Could you check a few things on this model? Use its own coordinates, in mm. A direction names the side the tool comes from. Coordinates: 2 decimals unless noted, no trailing zeros. Loops run counter-clockwise (first coordinate to the right, second up) from the corner with the lowest first, then second, coordinate; pieces in that order, holes last.
from build123d import *

# Parameters (mm, degrees)
SKETCH1_W             = 6.5
SKETCH1_H             = 3.5
BOSS_EXTRUDE1_DEPTH   = 1.6
CHAMFER1_SIZE         = 1
CHAMFER1_SIZE2        = 0.25
CHAMFER1_PART_2_SIZE  = 1
CHAMFER1_PART_2_SIZE2 = 0.25
CHAMFER1_PART_3_SIZE  = 1
CHAMFER1_PART_3_SIZE2 = 0.25
CHAMFER1_PART_4_SIZE  = 1
CHAMFER1_PART_4_SIZE2 = 0.25
CHAMFER2_SIZE         = 0.125
CHAMFER2_SIZE2        = 0.5
EXTRUDE_THIN1_DEPTH   = 1.5
EXTRUDE_THIN2_DEPTH   = 0.35
LPATTERN1_COUNT       = 3
LPATTERN1_PITCH       = 2.3


with BuildPart() as part:
    # Sketch1 → Boss-Extrude1 (new body)
    with BuildSketch(Plane(origin=(0, 0, 0), x_dir=(1, 0, 0), z_dir=(0, 1, 0))):
        Rectangle(SKETCH1_W, SKETCH1_H)
    extrude(amount=BOSS_EXTRUDE1_DEPTH)

    # Chamfer1
    chamfer1_edges = [part.edges().sort_by_distance(p)[0] for p in [
        (3.25, 1.6, 0),
    ]]
    chamfer1_side = [part.faces().sort_by_distance(p)[0] for p in [
        (3.25, 0.8, 0),
    ]]
    chamfer(chamfer1_edges, length=CHAMFER1_SIZE, length2=CHAMFER1_SIZE2, reference=chamfer1_side[0])

    # Chamfer1 part 2
    chamfer1_part_2_edges = [part.edges().sort_by_distance(p)[0] for p in [
        (0, 1.6, -1.75),
    ]]
    chamfer1_part_2_side = [part.faces().sort_by_distance(p)[0] for p in [
        (0, 0.8, -1.75),
    ]]
    chamfer(chamfer1_part_2_edges, length=CHAMFER1_PART_2_SIZE, length2=CHAMFER1_PART_2_SIZE2, reference=chamfer1_part_2_side[0])

    # Chamfer1 part 3
    chamfer1_part_3_edges = [part.edges().sort_by_distance(p)[0] for p in [
        (-3.25, 1.6, 0),
    ]]
    chamfer1_part_3_side = [part.faces().sort_by_distance(p)[0] for p in [
        (-3.25, 0.8, 0),
    ]]
    chamfer(chamfer1_part_3_edges, length=CHAMFER1_PART_3_SIZE, length2=CHAMFER1_PART_3_SIZE2, reference=chamfer1_part_3_side[0])

    # Chamfer1 part 4
    chamfer1_part_4_edges = [part.edges().sort_by_distance(p)[0] for p in [
        (0, 1.6, 1.75),
    ]]
    chamfer1_part_4_side = [part.faces().sort_by_distance(p)[0] for p in [
        (0, 0.8, 1.75),
    ]]
    chamfer(chamfer1_part_4_edges, length=CHAMFER1_PART_4_SIZE, length2=CHAMFER1_PART_4_SIZE2, reference=chamfer1_part_4_side[0])

    # Chamfer2
    chamfer2_edges = [part.edges().sort_by_distance(p)[0] for p in [
        (0, 0, -1.75),
        (3.25, 0, 0),
        (0, 0, 1.75),
        (-3.25, 0, 0),
    ]]
    chamfer2_side = [part.faces().sort_by_distance(p)[0] for p in [
        (0, 0, 0),
    ]]
    chamfer(chamfer2_edges, length=CHAMFER2_SIZE, length2=CHAMFER2_SIZE2, reference=chamfer2_side[0])

    # Sketch2 → Extrude-Thin1 (add, symmetric)
    with BuildSketch(Plane(origin=(0, 0, 0), x_dir=(0, 0, -1), z_dir=(1, 0, 0))):
        with BuildLine():
            Line((0, 0.69), (-2.25, 0.69))
            ThreePointArc((-2.25, 0.69), (-2.41838071, 0.656506994), (-2.561126984, 0.561126984))
            Line((-2.561126984, 0.561126984), (-2.836055715, 0.286198252))
            ThreePointArc((-2.836055715, 0.286198252), (-2.881573879, 0.254326091), (-2.935247882, 0.239944185))
            Line((-2.935247882, 0.239944185), (-3.512201804, 0.189467258))
            Line((-3.512201804, 0.189467258), (-3.487798196, -0.089467258))
            Line((-3.487798196, -0.089467258), (-2.910844274, -0.03899033))
            ThreePointArc((-2.910844274, -0.03899033), (-2.763240765, 0.000559911), (-2.638065817, 0.088208353))
            Line((-2.638065817, 0.088208353), (-2.363137085, 0.363137085))
            ThreePointArc((-2.363137085, 0.363137085), (-2.311229349, 0.397820725), (-2.25, 0.41))
            Line((-2.25, 0.41), (0, 0.41))
            Line((0, 0.41), (0, 0.69))
        make_face()
    extrude(amount=EXTRUDE_THIN1_DEPTH, both=True)

    # Sketch3 → Extrude-Thin2 (add, symmetric)
    with BuildSketch(Plane(origin=(2.3, 0, 0), x_dir=(0, 0, -1), z_dir=(1, 0, 0))):
        with BuildLine():
            Line((0, 0.41), (2.25, 0.41))
            ThreePointArc((2.25, 0.41), (2.311229349, 0.397820725), (2.363137085, 0.363137085))
            Line((2.363137085, 0.363137085), (2.638065817, 0.088208353))
            ThreePointArc((2.638065817, 0.088208353), (2.763240765, 0.000559911), (2.910844274, -0.03899033))
            Line((2.910844274, -0.03899033), (3.487798196, -0.089467258))
            Line((3.487798196, -0.089467258), (3.512201804, 0.189467258))
            Line((3.512201804, 0.189467258), (2.935247882, 0.239944185))
            ThreePointArc((2.935247882, 0.239944185), (2.881573879, 0.254326091), (2.836055715, 0.286198252))
            Line((2.836055715, 0.286198252), (2.561126984, 0.561126984))
            ThreePointArc((2.561126984, 0.561126984), (2.41838071, 0.656506994), (2.25, 0.69))
            Line((2.25, 0.69), (0, 0.69))
            Line((0, 0.69), (0, 0.41))
        make_face()
    extrude_thin2 = extrude(amount=EXTRUDE_THIN2_DEPTH, both=True)

    # LPattern1: Extrude-Thin2 ×3
    with Locations(*[(-i * LPATTERN1_PITCH, 0, 0) for i in range(1, LPATTERN1_COUNT)]):
        add(extrude_thin2)


solid = part.part
(1) Which directions (+Z, -Z, +X, -X, +Y, -Y) give clear straight access to the entire face, cutting with the end or side of a thin tool? Please do faces 1 (the face through (-3.123, 1.107, 0.024)), 2 (the face through (0, 0, 0)).
Answers:
face 1: +Z, -Z, -X, +Y
face 2: +X, -X, -Y
(2) I need wall thicknesses on probe 1 along Y at (x, z) = (-0.5, 0.25); probe 2 along Z at (x, y) = (0.75, 1.1) (3 decimals); probe 3 along X at (y, z) = (0.7, 0) (3 decimals). Which ranges of each line are inside material? Lowest first, please.
Answers:
probe 1: y = 0 to 1.6
probe 2: z = -1.625 to 1.625
probe 3: x = -3.225 to 3.225
(3) For pin 1 (0.6 mm diameter, centred on y = 0.5, z = -2.5, fed in from -X); pin 2 (1 mm diameter, centred on x = -0.5, y = 1, fed in from -Z); pin 3 (0.6 mm diameter, centred on y = 0, z = -2.5, fed in from +X), each with a flat end and sliding along its axis, tell me the tip position at first contact or that it passes through.
Answers:
pin 1: stops at x = -2.65
pin 2: stops at z = -2.6
pin 3: stops at x = 2.65
(4) Imagine slicing it at A-A, the plane z = -2. Write out the boundary of the cut face in (x, y).
Answers:
outline: (-2.65, 0.41) - (-1.95, 0.41) - (-1.95, 0.69) - (-2.65, 0.69) - close; (-0.35, 0.41) - (0.35, 0.41) - (0.35, 0.69) - (-0.35, 0.69) - close; (1.95, 0.41) - (2.65, 0.41) - (2.65, 0.69) - (1.95, 0.69) - close
(5) Imagine slicing it at C-C, the plane z = 0. Write out the boundary of the cut face in (x, y) (3 decimals), and give its area (3 significant figures).
Answers:
outline: (-3.25, 0.5) - (-3.125, 0) - (3.125, 0) - (3.25, 0.5) - (3.25, 0.6) - (3, 1.6) - (-3, 1.6) - (-3.25, 0.6) - close
area: 10.1 mm2
(6) Imagine slicing it at D-D, the plane y = 1. Write out the boundary of the cut face in (x, z), and give its area (3 significant figures).
Answers:
outline: (-3.15, -1.65) - (3.15, -1.65) - (3.15, 1.65) - (-3.15, 1.65) - close
area: 20.8 mm2
